The listing builds one solid part. Answer for the finished solid, in the listing's coordinates (mm). A direction names the side the tool comes from. Round coordinates to 2 decimals unless told otherwise and drop trailing zeros. Write each loop counter-clockwise with the first axis right and the second up, starting at its lowest first coordinate (ties: lowest second). Pieces come first, ordered by that corner, then holes.
(1) A cutting plane is placed at A-A, the plane y = 0.4. Give the vertices of the cut face in (x, z), and give its area (3 significant figures).
(2) Find the intervals of material crossed by probe 1 along X at (y, z) = (0.6, -330); probe 2 along X at (y, z) = (0.45, -60); probe 3 along X at (y, z) = (1.8, -64), in increasing order.
(3) For faces 1 (the face through (99, 0, -198)), 2 (the face through (129.594, 0.986, -32.719)), determine the directions among +Z, -Z, +X, -X, +Y, -Y from which every point of the face is accessible in a straight line to the end or side of a thin tool.
(4) Each of these flat-tipped pins is pushed along its axis until it touches: pin 1 Ø0.6 at (x, y) = (108, 0.5) entering from +Z; pin 2 Ø0.6 at (y, z) = (1, -379) entering from -X; pin 3 Ø0.6 at (x, y) = (29, 1) entering from -Z. Where does it stop, or does it pass through?
(5) A cutting plane is placed at B-B, the plane z = -48. Give the vertices of the cut face in (x, y), and give its area (3 significant figures).
from build123d import *

# Parameters (mm, degrees)
CROQUIS1_W              = 200
CROQUIS1_H              = 390
SALIENTE_EXTRUIR1_DEPTH = 2
CROQUIS3_W              = 55
CROQUIS3_H              = 30
CORTAR_EXTRUIR1_DEPTH   = 2
CROQUIS5_W              = 40
CROQUIS5_H              = 35
CORTAR_EXTRUIR3_DEPTH   = 2
CROQUIS6_W              = 35
CROQUIS6_H              = 125
CORTAR_EXTRUIR4_DEPTH   = 2
CROQUIS7_R              = 1.6
CORTAR_EXTRUIR5_DEPTH   = 2
REDONDEO1_R             = 8


with BuildPart() as part:
    # Croquis1 → Saliente-Extruir1 (new body)
    with BuildSketch(Plane(origin=(0, 0, 0), x_dir=(1, 0, 0), z_dir=(0, 1, 0))):
        with Locations((100, 195)):
            Rectangle(CROQUIS1_W, CROQUIS1_H)
    extrude(amount=SALIENTE_EXTRUIR1_DEPTH)

    # Croquis3 → Cortar-Extruir1 (cut)
    with BuildSketch(Plane(origin=(0, 2, 0), x_dir=(1, 0, 0), z_dir=(0, 1, 0))):
        with Locations((27.5, 375)):
            Rectangle(CROQUIS3_W, CROQUIS3_H)
        with Locations((27.5, 15)):
            Rectangle(CROQUIS3_W, CROQUIS3_H)
    extrude(amount=-CORTAR_EXTRUIR1_DEPTH, mode=Mode.SUBTRACT)

    # Croquis5 → Cortar-Extruir3 (cut)
    with BuildSketch(Plane(origin=(0, 2, 0), x_dir=(1, 0, 0), z_dir=(0, 1, 0))):
        with Locations((112, 17.5)):
            Rectangle(CROQUIS5_W, CROQUIS5_H)
    extrude(amount=-CORTAR_EXTRUIR3_DEPTH, mode=Mode.SUBTRACT)

    # Croquis6 → Cortar-Extruir4 (cut)
    with BuildSketch(Plane(origin=(0, 2, 0), x_dir=(1, 0, 0), z_dir=(0, 1, 0))):
        with Locations((182.5, 62.5)):
            Rectangle(CROQUIS6_W, CROQUIS6_H)
    extrude(amount=-CORTAR_EXTRUIR4_DEPTH, mode=Mode.SUBTRACT)

    # Croquis7 → Cortar-Extruir5 (cut)
    with BuildSketch(Plane(origin=(0, 2, 0), x_dir=(1, 0, 0), z_dir=(0, 1, 0))):
        with Locations(Location((15.05, 330, 0), (0, 0, 270))):
            Circle(CROQUIS7_R)
        with Locations(Location((15.05, 195, 0), (0, 0, 270))):
            Circle(CROQUIS7_R)
        with Locations(Location((15.05, 60, 0), (0, 0, 270))):
            Circle(CROQUIS7_R)
    extrude(amount=-CORTAR_EXTRUIR5_DEPTH, mode=Mode.SUBTRACT)

    # Redondeo1
    redondeo1_edges = [part.edges().sort_by_distance(p)[0] for p in [
        (55, 1, -360),
        (55, 1, -30),
        (132, 1, -35),
        (92, 1, -35),
        (165, 1, -125),
    ]]
    fillet(redondeo1_edges, radius=REDONDEO1_R)


solid = part.part
Solutions:
1. outline: (0, -360) - (47, -360) arc R8 cw to (55, -368) - (55, -390) - (200, -390) - (200, -125) - (173, -125) arc R8 cw to (165, -117) - (165, 0) - (132, 0) - (132, -27) arc R8 cw to (124, -35) - (100, -35) arc R8 cw to (92, -27) - (92, 0) - (55, 0) - (55, -22) arc R8 cw to (47, -30) - (0, -30) - close; hole circle Ø3.2 at (15.05, -330); hole circle Ø3.2 at (15.05, -195); hole circle Ø3.2 at (15.05, -60)
1. area: 69,000 mm2
2. probe 1: x = 0 to 13.45, 16.65 to 200
2. probe 2: x = 0 to 13.45, 16.65 to 165
2. probe 3: x = 0 to 165
3. face 1: +Z, -Z, +X, -X, -Y
3. face 2: +Z, +Y, -Y
4. pin 1: stops at z = -35
4. pin 2: stops at x = 55
4. pin 3: stops at z = -360
5. outline: (0, 0) - (165, 0) - (165, 2) - (0, 2) - close
5. area: 330 mm2
